Read the model definition and answer for the solid it produces. Units are mm, in the model's axes. A direction names the side the tool comes from. Coordinates: 2 decimals unless noted, no trailing zeros. Loops run counter-clockwise (first coordinate to the right, second up) from the corner with the lowest first, then second, coordinate; pieces in that order, holes last. Notation, with made-up numbers: M 5,89 L 42,89 A28 cw 42,116 Z; hole C 2.25,-35.75 d1. An arc over 180 degrees is marked long. Use one line per item in the form item = value. Start each with the question number.
1. The part is cut by section A-A (y = 0). Give the vertices of the cut face in (x, z), plus the area to 3 significant figures.
2. Find the intervals of material crossed by probe 1 along Y at (x, z) = (4, 3); probe 2 along Y at (x, z) = (0, 8.5); probe 3 along X at (y, z) = (10, 2.25), in increasing order. Write a range as [from, to].
3. The part is cut by section C-C (z = 7.75). Give the vertices of the cut face in (x, y).
4. For a pull along X with two mould halves and no side action, classify faces 1 (the cylindrical face through (47.69, 15.02, 8.92)), 2 (the cylindrical face through (-8.67, -39.05, 8.92)), 3 (the conical face through (-8.703, -39.191, 2.854)), 4 (the flat face through (-22, 34, 15)) as released by +X, released by -X, zero draft, split by the parting line, or undercut.
5. A tool of negligible diameter and unlimited length cuts with its end or side. For faces 5 (the flat face through (-26.2, 41, 15)), 6 (the flat face through (36, 22, 2)), from which of +Z, -Z, +X, -X, +Y, -Y can it reach the whole face along a straight path? Write none if from no direction.
6. Flat-ended cylindrical pins translate along their axes: pin 1 (4 mm diameter, centred on x = 35, z = 6, fed in from +Y); pin 2 (1 mm diameter, centred on y = -17.5, z = 13, fed in from -X); pin 3 (1 mm diameter, centred on y = -35.5, z = 11.5, fed in from +X); pin 4 (5 mm diameter, centred on x = -29, y = 32, fed in from -Z). Find the tip coordinate at first contact, or state that the pin passes through.
from build123d import *

# Parameters (mm, degrees)
F0_R     = 50
F0_R_2   = 40
F1_DEPTH = 15
F2_R     = 48.5
F2_R_2   = 41.5
F3_DEPTH = 13
F4_SIZE  = 3
F5_SIZE  = 3


with BuildPart() as f1:
    # F0 (on Top) → F1 (new body)
    with BuildSketch(Plane.XY):
        Circle(F0_R)
        Circle(F0_R_2, mode=Mode.SUBTRACT)
    extrude(amount=F1_DEPTH)

    # F2 (on face) → F3 (cut)
    with BuildSketch(Plane.XY.offset(15)):
        Circle(F2_R)
        Circle(F2_R_2, mode=Mode.SUBTRACT)
    extrude(amount=-F3_DEPTH, mode=Mode.SUBTRACT)

    # F4
    f4_edges = [f1.edges().sort_by_distance(p)[0] for p in [
        (-50, 0, 0),
    ]]
    chamfer(f4_edges, length=F4_SIZE)

    # F5
    f5_edges = [f1.edges().sort_by_distance(p)[0] for p in [
        (-40, 0, 0),
    ]]
    chamfer(f5_edges, length=F5_SIZE)


solid = f1.part
Computed values:
q1.outline = M -50,3 L -47,0 L -43,0 L -40,3 L -40,15 L -41.5,15 L -41.5,2 L -48.5,2 L -48.5,15 L -50,15 Z; M 40,3 L 43,0 L 47,0 L 50,3 L 50,15 L 48.5,15 L 48.5,2 L 41.5,2 L 41.5,15 L 40,15 Z
q1.area = 100 mm²
q2.probe_1 = [-49.84, -48.33], [-41.31, -39.8], [39.8, 41.31], [48.33, 49.84]
q2.probe_2 = [-50, -48.5], [-41.5, -40], [40, 41.5], [48.5, 50]
q2.probe_3 = [-48.22, -47.46], [-40.28, -39.5], [39.5, 40.28], [47.46, 48.22]
q3.outline = C 0,0 d100; C 0,0 d83; hole C 0,0 d97; hole C 0,0 d80
q4.face_1 = split by the parting line
q4.face_2 = undercut
q4.face_3 = undercut
q4.face_4 = zero draft
q5.face_5 = +Z, +X, -X, +Y, -Y
q5.face_6 = +Z
q6.pin_1 = 37.56
q6.pin_2 = -47.02
q6.pin_3 = 35.71
q6.pin_4 = 0
